```python
from build123d import *

# Parameters (mm, degrees)
BOSS_EXTRUDE1_DEPTH = 50
FILLET1_R           = 2


with BuildPart() as part:
    # Sketch1 → Boss-Extrude1 (new body)
    with BuildSketch(Plane.XY):
        Polygon((410, 480), (410, 50), (50, 50), (50, 480), (0, 480), (0, 50), (0, 0), (460, 0), (460, 50), (460, 480), align=None)
    extrude(amount=BOSS_EXTRUDE1_DEPTH)

    # Fillet1
    fillet1_edges = [part.edges().sort_by_distance(p)[0] for p in [
        (460, 240, 0),
        (230, 0, 0),
        (0, 240, 0),
        (50, 265, 0),
        (0, 240, 50),
        (460, 240, 50),
        (230, 50, 50),
        (50, 265, 50),
        (230, 50, 0),
        (410, 265, 0),
    ]]
    fillet(fillet1_edges, radius=FILLET1_R)


solid = part.part
```
Build history of the part. All positions in model axes, mm. A direction names the side the tool comes from. Round coordinates to 2 decimals unless told otherwise and drop trailing zeros. Write each loop counter-clockwise with the first axis right and the second up, starting at its lowest first coordinate (ties: lowest second). Pieces come first, ordered by that corner, then holes. Notation, with made-up numbers: (34.25, 23) - (48.25, 23) arc R24 ccw to (48.25, 40) - close; hole circle Ø10 at (51, 6.25). An arc over 180 degrees is marked (long way). Write each question's results on one line, items separated by ' | '. Start each with the question number.
Item 1: Mould opens along X. For faces 3 (the face through (25, 480, 25)), 4 (the face through (0, 243, 25)), 5 (the face through (410, 267, 26)), 6 (the face through (460, 237, 25)) say: pulls with the +X half, pulls with the -X half, needs draft (parallel to the pull), parting line crosses it, or undercut.
Item 2: Which spindle directions (+Z, -Z, +X, -X, +Y, -Y) get a long thin tool onto all of the face, cutting with end or side? Do faces 1 (the face through (233, 50, 25)), 2 (the face through (435, 480, 25)). Say none if no direction does.
Item 3: Saw through at C-C (x = 152.5). Write the cut outline in (y, z).
Item 4: Drop flat-ended pins along their axis: P1, Ø5, axis at x = 399, y = 53, coming from the +Z side; P2, Ø3, axis at x = 295.5, z = 24.5, coming from the +Y side. Give the stop position or say it passes through.
Item 5: Saw through at B-B (z = 25.5). Write the cut outline in (x, y), and give its area (3 significant figures).
Item 6: Wall check: L1, parallel to X at y = 137.5, z = 29; L2, parallel to Y at x = 258, z = 21; L3, parallel to Y at x = 211.5, z = 48.5. Give the ranges that are in metal, low to high. Write a range as [from, to].
Item 7: Saw through at A-A (y = 112.5). Write the cut outline in (x, z).
Results are:
1) face 3: needs draft | face 4: pulls with the -X half | face 5: undercut | face 6: pulls with the +X half
2) face 1: +Z, -Z, +Y | face 2: +Z, -Z, +X, -X, +Y
3) outline: (0, 2) arc R2 ccw to (2, 0) - (48, 0) arc R2 ccw to (50, 2) - (50, 48) arc R2 ccw to (48, 50) - (0, 50) - close
4) P1: passes through | P2: stops at y = 50
5) outline: (0, 0) - (460, 0) - (460, 480) - (410, 480) - (410, 50) - (50, 50) - (50, 480) - (0, 480) - close | area: 66,000 mm²
6) L1: x = [0, 50], [410, 460] | L2: y = [0, 50] | L3: y = [0, 49.94]
7) outline: (0, 2) arc R2 ccw to (2, 0) - (48, 0) arc R2 ccw to (50, 2) - (50, 48) arc R2 ccw to (48, 50) - (2, 50) arc R2 ccw to (0, 48) - close; (410, 2) arc R2 ccw to (412, 0) - (458, 0) arc R2 ccw to (460, 2) - (460, 48) arc R2 ccw to (458, 50) - (410, 50) - close
